```python
from build123d import *

# Parameters (mm, degrees)
EXTRUDE_1_DEPTH          = 15
CUT_EXTRUDE_1_DEPTH      = 109.392019307
CUT_EXTRUDE_1_DEPTH_BACK = 109.392019307
SKETCH_3_R               = 30
SKETCH_3_3_R             = 30
EXTRUDE_2_DEPTH          = 15
EXTRUDE_3_DEPTH          = 15
CUT_EXTRUDE_2_DEPTH      = 153.192153917
CUT_EXTRUDE_2_DEPTH_BACK = 153.192153917
FILLET_1_R               = 5
FILLET_2_R               = 2


with BuildPart() as part:
    # 草图1 → 凸台-拉伸1 (new, symmetric)
    with BuildSketch(Plane.XY):
        Polygon((0, 0), (80, 0), (106.830127019, -15.490381057), (114.330127019, -2.5), (84.019237886, 15), (3.32541994, 15), (-25.38149862, 28.386255966), (-31.720772546, 14.791639161), align=None)
    extrude(amount=EXTRUDE_1_DEPTH, both=True)

    # 草图3 → 切除-拉伸1 (cut, two sides: drawn at the far end of the back side and taken through both)
    with BuildSketch(Plane(origin=(27.5, 47.631397208, 0), x_dir=(0.866025403784438, -0.5000000000000012, 0), z_dir=(0.5000000000000012, 0.866025403784438, 0)).offset(-CUT_EXTRUDE_1_DEPTH_BACK)):
        with Locations((104.345320277, 0)):
            Circle(SKETCH_3_R)
        Polygon((119.345320277, -6.213203436), (119.345320277, 6.213203436), (110.558523712, 15), (98.132116841, 15), (89.345320277, 6.213203436), (89.345320277, -6.213203436), (98.132116841, -15), (110.558523712, -15), align=None, mode=Mode.SUBTRACT)
    extrude(amount=CUT_EXTRUDE_1_DEPTH + CUT_EXTRUDE_1_DEPTH_BACK, mode=Mode.SUBTRACT)


with BuildPart() as body_2:
    # of the pieces the cut leaves, the one that is kept (cut_extrude_1_keep)
    add(part.part.solids().sort_by_distance((0, 0, -15))[0])

    # 草图3<3> → 凸台-拉伸2 (add)
    with BuildSketch(Plane(origin=(27.5, 47.631397208, 0), x_dir=(0.866025403784438, -0.5000000000000012, 0), z_dir=(0.5000000000000012, 0.866025403784438, 0))):
        with Locations((104.345320277, 0)):
            Circle(SKETCH_3_3_R)
        Polygon((119.345320277, -6.213203436), (119.345320277, 6.213203436), (110.558523712, 15), (98.132116841, 15), (89.345320277, 6.213203436), (89.345320277, -6.213203436), (98.132116841, -15), (110.558523712, -15), align=None, mode=Mode.SUBTRACT)
    extrude(amount=-EXTRUDE_2_DEPTH)

    # 草图6 → 凸台-拉伸3 (add)
    with BuildSketch(Plane(origin=(0, 0, 0), x_dir=(0.9063077870366528, -0.4226182617406936, 0), z_dir=(-0.4226182617406936, -0.9063077870366528, 0))):
        with BuildLine():
            Line((-61.608269391, 13.856406461), (-35, 13.856406461))
            Line((-35, 13.856406461), (-35, 15))
            Line((-35, 15), (-9.019237886, 15))
            ThreePointArc((-9.019237886, 15), (-35.652221505, 29.99290928), (-61.608269391, 13.856406461))
        make_face()
        with BuildLine():
            Line((-35, 15), (-35, 13.856406461))
            Line((-35, 13.856406461), (-23, 6.92820323))
            Line((-23, 6.92820323), (-23, -6.92820323))
            Line((-23, -6.92820323), (-35, -13.856406461))
            Line((-35, -13.856406461), (-35, -15))
            Line((-35, -15), (-9.019237886, -15))
            ThreePointArc((-9.019237886, -15), (-5, 0), (-9.019237886, 15))
            Line((-9.019237886, 15), (-35, 15))
        make_face()
        with BuildLine():
            Line((-35, -15), (-35, -13.856406461))
            Line((-35, -13.856406461), (-61.608269391, -13.856406461))
            ThreePointArc((-61.608269391, -13.856406461), (-35.652221505, -29.99290928), (-9.019237886, -15))
            Line((-9.019237886, -15), (-35, -15))
        make_face()
    extrude(amount=-EXTRUDE_3_DEPTH)

    # 草图6<4> → 切除-拉伸2 (cut, two sides: drawn at the far end of the back side and taken through both)
    with BuildSketch(Plane(origin=(0, 0, 0), x_dir=(0.9063077870366528, -0.4226182617406936, 0), z_dir=(-0.4226182617406936, -0.9063077870366528, 0)).offset(-CUT_EXTRUDE_2_DEPTH_BACK)):
        Polygon((-23, 6.92820323), (-35, 13.856406461), (-35, -13.856406461), (-23, -6.92820323), align=None)
    extrude(amount=CUT_EXTRUDE_2_DEPTH + CUT_EXTRUDE_2_DEPTH_BACK, mode=Mode.SUBTRACT)

    # 圆角1
    fillet_1_edges = [body_2.edges().sort_by_distance(p)[0] for p in [
        (-5.004568567, 10.609003041, -15),
        (-5.004568567, 10.609003041, 15),
    ]]
    fillet(fillet_1_edges, radius=FILLET_1_R)

    # 圆角2
    fillet_2_edges = [body_2.edges().sort_by_distance(p)[0] for p in [
        (-52.666417332, 32.834088122, -13.856406461),
        (-52.666417332, 32.834088122, 13.856406461),
    ]]
    fillet(fillet_2_edges, radius=FILLET_2_R)


solid = body_2.part
```
Can you work these out from the model? Positions are in its coordinate system, mm. A direction names the side the tool comes from. Coordinates: 2 decimals unless noted, no trailing zeros. Order: outer loops, then holes, each group sorted by start corner. A loop starts at its lowest first (then second) coordinate and runs counter-clockwise, first axis right, second up.
1. Thinking about a two-plate mould opening in X: for faces 4 (the face through (101.178, -3.446, -0.087)), 5 (the face through (105.04, -5.67, -10.67)), 6 (the face through (39, 0, 0)), which applies, +X half, -X half, draft (parallel to the pull), parting line (faces both ways), or undercut?
2. I need wall thicknesses on line 1 (X direction, y = 5, z = -18); line 2 (Z direction, x = 43, y = 1.5); line 3 (Y direction, x = 35.5, z = -8). Which ranges of each line are inside material? Lowest first, please.
3. If we section it at A-A (z = 2): Please give me the cut outline in (x, y), then the cut area to 3 significant figures.
4. If we section it at B-B (x = 47.5): Please give me the cut outline in (y, z).
5. For faces 1 (the face through (114, -11, 15)), 2 (the face through (-39, 26, -13.856)), 3 (the face through (104.929, -5.611, 10.545)), which set-ups out of +Z, -Z, +X, -X, +Y, -Y let a thin tool reach every point of the face, with its end or its side?
6. If we section it at D-D (z = 25): Please give me the cut outline in (x, y), then the cut area to 3 significant figures.
7. If we section it at C-C (z = -9.5): Please give me the cut outline in (x, y).
8. I'm going to push flat-ended pins straight in: pin 1 (1 mm diameter, centred on x = 116.5, z = -15, fed in from -Y); pin 2 (6 mm diameter, centred on x = 27.5, y = 4, fed in from +Z); pin 3 (6 mm diameter, centred on x = 97.5, z = -21.5, fed in from -Y); pin 4 (12 mm diameter, centred on x = 117, y = -17, fed in from +Z). Where does each tip first touch, or does it pass through?
Entries:
1. face 4: +X half
1. face 5: undercut
1. face 6: draft
2. line 1: x = -10.72 to -9.81, 95.66 to 101.34
2. line 2: z = -15 to 15
2. line 3: y = 0 to 15
3. outline: (-20.85, 9.72) - (0, 0) - (80, 0) - (97.38, -10.03) - (104.88, 2.96) - (84.02, 15) - (3.33, 15) - (-14.51, 23.31) - close; (123.36, -25.03) - (136.29, -32.5) - (143.79, -19.51) - (130.86, -12.04) - close
3. area: 2,080 mm2
4. outline: (0, -15) - (15, -15) - (15, 15) - (0, 15) - close
5. face 1: none
5. face 2: -X, +Y
5. face 3: -Y
6. outline: (-46.75, 21.8) - (-16.69, 7.78) - (-10.35, 21.38) - (-40.41, 35.39) - close; (96, -9.24) - (124.73, -25.82) - (132.23, -12.83) - (103.5, 3.75) - close
6. area: 995 mm2
7. outline: (-24.88, 11.6) - (0, 0) - (80, 0) - (100.22, -11.68) - (107.72, 1.32) - (84.02, 15) - (3.33, 15) - (-18.54, 25.2) - close; (120.51, -23.39) - (135.01, -31.76) - (142.51, -18.77) - (128.01, -10.4) - close
8. pin 1: stops at y = -21.36
8. pin 2: stops at z = 15
8. pin 3: stops at y = -11.84
8. pin 4: stops at z = 30
